Check sheet for the modelled part. Datum: model origin and axes. Units: mm. Face numbers are marked on the shaded views. A direction names the side the tool comes from. Give positions to 0.01 mm unless a question says otherwise; leave off trailing zeros. Write each loop counter-clockwise with the first axis right and the second up, starting at its lowest first coordinate (ties: lowest second). Pieces come first, ordered by that corner, then holes. Notation, with made-up numbers: M -20,52 L 3,52 A14 ccw 3,61 Z; hole C -14,-11.5 d1. An arc over 180 degrees is marked long. Write item = value, one per line. Start each with the question number.
1) Access from +Z, -Z, +X, -X, +Y, -Y to the whole of each face (thin tool, end or side, straight path). Record for the marked faces 5 and 6.
2) Cross-section at D-D, the plane y = -2.25. Record the cut outline in (x, z).
3) Go/stop test with a flat-tipped pin: pin 1 (2.5 mm diameter, centred on y = -8, z = 92, fed in from +X). Record where the tip stops, or that it passes through.
4) Scan lines: line 1 along Y through (x, z) = (0.8, 92); line 2 along Y through (x, z) = (-0.95, 102.25); line 3 along Y through (x, z) = (1.2, 91.25). Record each from-to range of solid material in increasing order. Write a range as [from, to].
5) Cross-section at B-B, the plane z = 102.5. Record the cut outline in (x, y).
6) Mould release check, pull along Y, two halves, no side actions. Record for the marked faces 1, 2, 3 and 4: released by +Y, released by -Y, zero draft, split by the parting line, or undercut.
7) Cross-section at C-C, the plane y = -8.25. Record the cut outline in (x, z), plus the area to 3 significant figures.
8) Cross-section at A-A, the plane x = 0.55. Record the cut outline in (y, z).
```python
from build123d import *

# Parameters (mm, degrees)
SKETCH_1_R      = 1.55
EXTRUDE_1_DEPTH = 1.5
FILLET_1_R      = 3


with BuildPart() as part:
    # 草图1 → 凸台-拉伸1 (new body, symmetric)
    with BuildSketch(Plane(origin=(0, 0, 0), x_dir=(0, 0, -1), z_dir=(1, 0, 0))):
        with BuildLine():
            Line((-89, 11), (-89, -11))
            Line((-89, -11), (-110, -11))
            Line((-110, -11), (-110, -5))
            Line((-110, -5), (-107, -2))
            Line((-107, -2), (-99, -2))
            ThreePointArc((-99, -2), (-97, 0), (-99, 2))
            Line((-99, 2), (-107, 2))
            Line((-107, 2), (-110, 5))
            Line((-110, 5), (-110, 11))
            Line((-110, 11), (-89, 11))
        make_face()
        with Locations((-107, 8)):
            Circle(SKETCH_1_R, mode=Mode.SUBTRACT)
        with Locations((-92, 8)):
            Circle(SKETCH_1_R, mode=Mode.SUBTRACT)
        with Locations((-92, -8)):
            Circle(SKETCH_1_R, mode=Mode.SUBTRACT)
        with Locations((-107, -8)):
            Circle(SKETCH_1_R, mode=Mode.SUBTRACT)
    extrude(amount=EXTRUDE_1_DEPTH, both=True)

    # 圆角1
    fillet_1_edges = [part.edges().sort_by_distance(p)[0] for p in [
        (0, 11, 110),
        (0, 11, 89),
        (0, -11, 89),
        (0, -11, 110),
    ]]
    fillet(fillet_1_edges, radius=FILLET_1_R)


solid = part.part
```
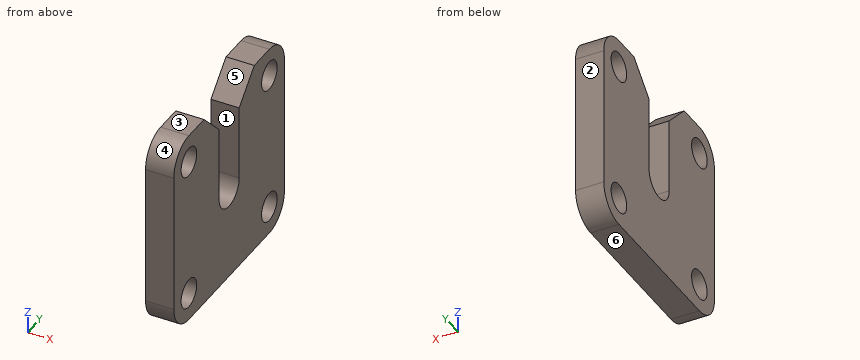
Reply:
q1.face_5 = +Z, +X, -X
q1.face_6 = -Z, +X, -X, +Y, -Y
q2.outline = M -1.5,89 L 1.5,89 L 1.5,107.25 L -1.5,107.25 Z
q3.pin_1 = through
q4.line_1 = [-11, -9.55], [-6.45, 6.45], [9.55, 11]
q4.line_2 = [-11, -2], [2, 11]
q4.line_3 = [-10.9, -9.36], [-6.64, 6.64], [9.36, 10.9]
q5.outline = M -1.5,-11 L 1.5,-11 L 1.5,-2 L -1.5,-2 Z; M -1.5,2 L 1.5,2 L 1.5,11 L -1.5,11 Z
q6.face_1 = undercut
q6.face_2 = released by +Y
q6.face_3 = zero draft
q6.face_4 = released by -Y
q7.outline = M -1.5,89.01 L 1.5,89.01 L 1.5,90.47 L -1.5,90.47 Z; M -1.5,93.53 L 1.5,93.53 L 1.5,105.47 L -1.5,105.47 Z; M -1.5,108.53 L 1.5,108.53 L 1.5,109.99 L -1.5,109.99 Z
q7.area = 44.6 mm2
q8.outline = M -11,92 A3 ccw -8,89 L 8,89 A3 ccw 11,92 L 11,107 A3 ccw 8,110 L 5,110 L 2,107 L 2,99 A2 cw -2,99 L -2,107 L -5,110 L -8,110 A3 ccw -11,107 Z; hole C -8,92 d3.1; hole C -8,107 d3.1; hole C 8,92 d3.1; hole C 8,107 d3.1
